```python
from build123d import *

# Parameters (mm, degrees)
F0_W     = 10
F0_H     = 12
F1_DEPTH = 2.5
F2_R     = 2.5
F2_R_2   = 0.5
F3_DEPTH = 4
F4_R     = 0.5


with BuildPart() as f1:
    # F0 (on Front) → F1 (new body, symmetric)
    with BuildSketch(Plane.XZ):
        Rectangle(F0_W, F0_H)
    extrude(amount=F1_DEPTH, both=True)

    # F2 (on face) → F3 (cut)
    with BuildSketch(Plane.XZ.offset(2.5)):
        with Locations((0, 2)):
            Circle(F2_R)
        with Locations((0, 2)):
            Circle(F2_R_2, mode=Mode.SUBTRACT)
    extrude(amount=-F3_DEPTH, mode=Mode.SUBTRACT)

    # F4
    f4_edges = [f1.edges().sort_by_distance(p)[0] for p in [
        (-0.5, -2.5, 2),
    ]]
    fillet(f4_edges, radius=F4_R)


solid = f1.part
```
Part model, mm, in its own coordinate system. A direction names the side the tool comes from. Round coordinates to 2 decimals unless told otherwise and drop trailing zeros. Loops run counter-clockwise (first coordinate to the right, second up) from the corner with the lowest first, then second, coordinate; pieces in that order, holes last.
1. Slice it at A-A (y = 0.4). Give the cut face in (x, z), and give its area (3 significant figures).
Solutions:
outline: (-5, -6) - (5, -6) - (5, 6) - (-5, 6) - close; circle Ø1 at (0, 2); hole circle Ø5 at (0, 2)
area: 101 mm2
2. Drill centre lines: line 1 along Z through (x, y) = (0, -0.15); line 2 along Y through (x, z) = (0.5, 1.5); line 3 along X through (y, z) = (-1.7, 0). Where is each one in solid material? Low to high.
Solutions:
line 1: z = -6 to -0.5, 1.5 to 2.5, 4.5 to 6
line 2: y = 1.5 to 2.5
line 3: x = -5 to -1.5, 1.5 to 5
3. 3-axis set-ups, long thin cutter, end or side, ignore diameter. For faces 1 (the face through (0, 2.5, 0)), 2 (the face through (0, 1.5, 1)): which of +Z, -Z, +X, -X, +Y, -Y reach the whole face in a straight line?
Solutions:
face 1: +Z, -Z, +X, -X, +Y
face 2: -Y
4. Slice it at C-C (x = 0). Give the cut face in (y, z).
Solutions:
outline: (-2.5, -6) - (2.5, -6) - (2.5, 6) - (-2.5, 6) - (-2.5, 4.5) - (1.5, 4.5) - (1.5, 2.5) - (-2, 2.5) arc R0.5 ccw to (-2, 1.5) - (1.5, 1.5) - (1.5, -0.5) - (-2.5, -0.5) - close
5. Slice it at D-D (x = 1.5). Give the cut face in (y, z), and give its area (3 significant figures).
Solutions:
outline: (-2.5, -6) - (2.5, -6) - (2.5, 6) - (-2.5, 6) - (-2.5, 4) - (1.5, 4) - (1.5, 0) - (-2.5, 0) - close
area: 44.0 mm2
6. Slice it at B-B (z = 2). Give the cut face in (x, y), and give its area (3 significant figures).
Solutions:
outline: (-5, -2.5) - (-2.5, -2.5) - (-2.5, 1.5) - (-0.5, 1.5) - (-0.5, -2) arc R0.5 ccw to (0.5, -2) - (0.5, 1.5) - (2.5, 1.5) - (2.5, -2.5) - (5, -2.5) - (5, 2.5) - (-5, 2.5) - close
area: 33.9 mm2
7. Two-plate mould, pull along X, no slides. Class faces 3 (the face through (-0.065, -0.274, 2.496)), 4 (the face through (-5, 0, 0)), 5 (the face through (5, 0, 0)), 6 (the face through (0, 0, -6)): pulls with the +X half, pulls with the -X half, needs draft (parallel to the pull), parting line crosses it, or undercut.
Solutions:
face 3: undercut
face 4: pulls with the -X half
face 5: pulls with the +X half
face 6: needs draft
